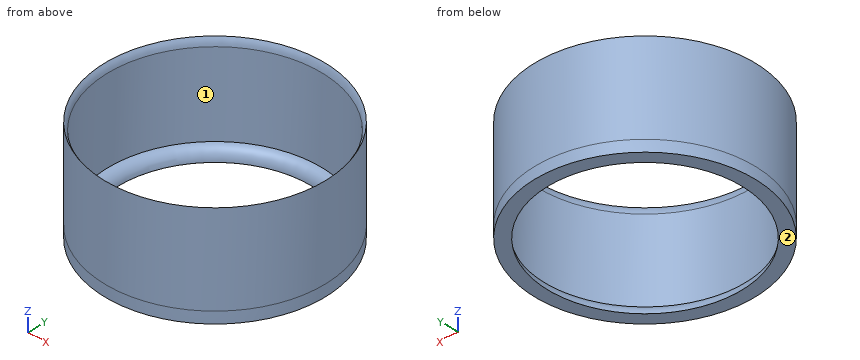
```python
from build123d import *

# Parameters (mm, degrees)
CROQUIS1_R              = 482.5
CROQUIS1_R_2            = 470
SALIENTE_EXTRUIR1_DEPTH = 400
REDONDEO1_R             = 50
SALIENTE_EXTRUIR2_START = 50
CROQUIS2_R              = 482.5
CROQUIS2_R_2            = 425
SALIENTE_EXTRUIR2_DEPTH = 50
REDONDEO3_R             = 50


with BuildPart() as part:
    # Croquis1 → Saliente-Extruir1 (new body)
    with BuildSketch(Plane(origin=(0, 0, 0), x_dir=(0, 1, 0), z_dir=(0, 0, 1))):
        with Locations(Location((0, 0, 0), (0, 0, 270))):
            Circle(CROQUIS1_R)
        with Locations(Location((0, 0, 0), (0, 0, 270))):
            Circle(CROQUIS1_R_2, mode=Mode.SUBTRACT)
    extrude(amount=SALIENTE_EXTRUIR1_DEPTH)

    # Redondeo1
    # the kernel refuses this fillet: 50 mm, written as the material it takes off along each edge
    with BuildSketch(Plane(origin=(0, 0, 400), x_dir=(1, 0, 0), z_dir=(0, -1, 0))) as redondeo1_piece_1:
        with BuildLine():
            CenterArc((520, -33.071891388), REDONDEO1_R, 138.590377891, 41.409622109)
            Line((482.5, 0), (481.75, 0.661437828))
            ThreePointArc((481.75, 0.661437828), (476.25, 1), (470, 1))
            Line((470, 1), (469, 0))
            Line((469, 0), (469, -33.071891388))
            Line((469, -33.071891388), (470, -33.071891388))
        make_face()
    revolve(axis=Axis((0, 0, 400), (0, 0, 1)), mode=Mode.SUBTRACT)

    # Croquis2 → Saliente-Extruir2 (add)
    with BuildSketch(Plane(origin=(0, 0, 0), x_dir=(1, 0, 0), z_dir=(0, 0, -1)).offset(SALIENTE_EXTRUIR2_START)):
        with Locations(Location((0, 0, 0), (0, 0, 180))):
            Circle(CROQUIS2_R)
        with Locations(Location((0, 0, 0), (0, 0, 180))):
            Circle(CROQUIS2_R_2, mode=Mode.SUBTRACT)
    extrude(amount=-SALIENTE_EXTRUIR2_DEPTH)

    # Redondeo3
    # the kernel refuses this fillet: 50 mm, written as the material it takes off along each edge
    with BuildSketch(Plane(origin=(0, 0, 0), x_dir=(-1, 0, 0), z_dir=(0, -1, 0))) as redondeo3_piece_1:
        with BuildLine():
            CenterArc((475, 49.749371855), REDONDEO3_R, 180, 84.260829523)
            Line((470, 0), (469.9, -0.994987437))
            ThreePointArc((469.9, -0.994987437), (447.5, -1), (425, -1))
            Line((425, -1), (424, 0))
            Line((424, 0), (424, 49.749371855))
            Line((424, 49.749371855), (425, 49.749371855))
        make_face()
    revolve(axis=Axis((0, 0, 0), (0, 0, -1)), mode=Mode.SUBTRACT)


solid = part.part
```
For this review, take the finished solid that the model builds, in its own axes (mm). Face numbers are marked on the shaded views. Coordinates: 2 decimals unless noted, no trailing zeros. Loops run counter-clockwise (first coordinate to the right, second up) from the corner with the lowest first, then second, coordinate; pieces in that order, holes last. Notation, with made-up numbers: (66.5, -3.5) -> (80.5, -3.5) arc R8 ccw to (80.5, 3.5) -> close; hole circle Ø6 at (-19, 74.25). An arc over 180 degrees is marked (long way). Return JSON: item names as keys, results as strings. Group by question number.
(1) Mouldability with a two-part tool opening along X and no side actions: class the marked faces 1 and 2 as pulls with the +X half, pulls with the -X half, needs draft (parallel to the pull), parting line crosses it, or undercut.
(2) Consider section C-C, the plane z = 260.5. Give the boundary of the cut face in (x, y), plus the area to 3 significant figures.
(3) To check wall thickness, follow L1, parallel to X at y = 0, z = 166.5; L2, parallel to Y at x = 0, z = -49.9. State the ranges of each line that lie inside material, in increasing order.
(4) For pin 1 Ø12 at (y, z) = (-382.5, 110.5) entering from +X; pin 2 Ø1.5 at (y, z) = (321, 37) entering from -X; pin 3 Ø12 at (x, z) = (333, 202.5) entering from -Y, all flat-tipped, find the tip position at first contact; note any pin that passes through.
(5) Consider section A-A, the plane x = 0. Give the boundary of the cut face in (y, z), plus the area to 3 significant figures.
Results below:
{
 "1": {"face 1": "undercut", "face 2": "needs draft"},
 "2": {"outline": "circle Ø965 at (0, 0); hole circle Ø940 at (0, 0)", "area": "37,400 mm2"},
 "3": {"L1": "x = -482.5 to -470, 470 to 482.5", "L2": "y = -482.5 to -425, 425 to 482.5"},
 "4": {"pin 1": "stops at x = 301.75", "pin 2": "stops at x = -360.9", "pin 3": "stops at y = -354.79"},
 "5": {"outline": "(-482.5, -50) -> (-425, -50) -> (-425, -49.75) arc R50 ccw to (-470, 0) -> (-470, 366.93) arc R50 ccw to (-482.5, 400) -> close; (425, -50) -> (482.5, -50) -> (482.5, 400) arc R50 ccw to (470, 366.93) -> (470, 0) arc R50 ccw to (425, -49.75) -> close", "area": "14,400 mm2"}
}
